```python
from build123d import *

# Parameters (mm, degrees)
SKETCH1_R           = 32.5
SKETCH1_R_2         = 2.3
SKETCH1_R_3         = 1.7
BOSS_EXTRUDE1_DEPTH = 5


with BuildPart() as part:
    # Sketch1 → Boss-Extrude1 (new body)
    with BuildSketch(Plane(origin=(0, 0, 0), x_dir=(1, 0, 0), z_dir=(0, 1, 0))):
        with Locations(Location((0, 0, 0), (0, 0, 270))):
            Circle(SKETCH1_R)
        with Locations(Location((-15, 20, 0), (0, 0, 270))):
            Circle(SKETCH1_R_2, mode=Mode.SUBTRACT)
        with Locations(Location((-22.5, 15, 0), (0, 0, 270))):
            Circle(SKETCH1_R_3, mode=Mode.SUBTRACT)
        with Locations(Location((-15, -20, 0), (0, 0, 270))):
            Circle(SKETCH1_R_2, mode=Mode.SUBTRACT)
        with Locations(Location((-25, 0, 0), (0, 0, 270))):
            Circle(SKETCH1_R_2, mode=Mode.SUBTRACT)
        with Locations(Location((-22.5, -15, 0), (0, 0, 270))):
            Circle(SKETCH1_R_3, mode=Mode.SUBTRACT)
        with Locations(Location((15, -20, 0), (0, 0, 90))):
            Circle(SKETCH1_R_2, mode=Mode.SUBTRACT)
        with Locations(Location((22.5, -15, 0), (0, 0, 90))):
            Circle(SKETCH1_R_3, mode=Mode.SUBTRACT)
        with Locations(Location((25, 0, 0), (0, 0, 90))):
            Circle(SKETCH1_R_2, mode=Mode.SUBTRACT)
        with Locations(Location((22.5, 15, 0), (0, 0, 90))):
            Circle(SKETCH1_R_3, mode=Mode.SUBTRACT)
        with Locations(Location((15, 20, 0), (0, 0, 90))):
            Circle(SKETCH1_R_2, mode=Mode.SUBTRACT)
        with BuildLine():
            Line((-9, 6.168261928), (-9, -16.9))
            Line((-9, -16.9), (9, -16.9))
            Line((9, -16.9), (9, 6.168261928))
            ThreePointArc((9, 6.168261928), (0, 19.3), (-9, 6.168261928))
        make_face(mode=Mode.SUBTRACT)
        with BuildLine():
            ThreePointArc((7.695243167, 22.633068138), (10.866931862, 24.195243167), (9.304756833, 27.366931862))
            ThreePointArc((9.304756833, 27.366931862), (0, 28.905491853), (-9.304756833, 27.366931862))
            ThreePointArc((-9.304756833, 27.366931862), (-10.866931862, 24.195243167), (-7.695243167, 22.633068138))
            ThreePointArc((-7.695243167, 22.633068138), (0, 23.905491853), (7.695243167, 22.633068138))
        make_face(mode=Mode.SUBTRACT)
        with BuildLine():
            ThreePointArc((7.695243167, -22.633068138), (10.866931862, -24.195243167), (9.304756833, -27.366931862))
            ThreePointArc((9.304756833, -27.366931862), (0, -28.905491853), (-9.304756833, -27.366931862))
            ThreePointArc((-9.304756833, -27.366931862), (-10.866931862, -24.195243167), (-7.695243167, -22.633068138))
            ThreePointArc((-7.695243167, -22.633068138), (0, -23.905491853), (7.695243167, -22.633068138))
        make_face(mode=Mode.SUBTRACT)
    extrude(amount=BOSS_EXTRUDE1_DEPTH)


solid = part.part
```
Source: CAD feature listing. Evaluate the final solid. Frame: model axes, mm. Give positions to 0.01 mm unless a question says otherwise; leave off trailing zeros. Order: outer loops, then holes, each group sorted by start corner. A loop starts at its lowest first (then second) coordinate and runs counter-clockwise, first axis right, second up.
(1) Section query C-C (x = -1.5). Return the cut outline in (y, z), plus the area to 3 significant figures.
(2) Contact query for flat-ended pins moving along their axis: P1, Ø4, axis at x = 15, z = -20, coming from the +Y side; P2, Ø2.5, axis at y = 1.5, z = 0, coming from the +X side; P3, Ø1.5, axis at y = 2.5, z = 3, coming from the -X side; P4, Ø1, axis at x = 17, y = 1, coming from the -Z side. Output: stop coordinate, or through.
(3) Pull-direction query (Z, two-part tool) for faces 1 (the face through (9, 2, 6)), 2 (the face through (9.76, 2.46, 31)), 3 (the face through (-14, 0, 0)); classes: +Z half, -Z half, draft (parallel to the pull), parting line (faces both ways), or undercut.
(4) Material intervals for line 1 along X through (y, z) = (2.15, 0); line 2 along Z through (x, y) = (1.5, 2.45); line 3 along Z through (x, y) = (7.5, 4.25), sorted ascending.
(5) Section query A-A (y = 3.25). State how many separate pieces and enclosed holes the cut face has, plus the area to 3 significant figures.
(6) Section query D-D (z = -9.65). Return the cut outline in (x, y).
(7) Section query B-B (z = 0). Return the cut outline in (x, y).
Outcome:
1. outline: (0, -32.47) - (5, -32.47) - (5, -28.87) - (0, -28.87) - close; (0, -23.86) - (5, -23.86) - (5, -19.18) - (0, -19.18) - close; (0, 16.9) - (5, 16.9) - (5, 23.86) - (0, 23.86) - close; (0, 28.87) - (5, 28.87) - (5, 32.47) - (0, 32.47) - close
1. area: 94.2 mm2
2. P1: passes through
2. P2: stops at x = 32.5
2. P3: stops at x = -32.42
2. P4: stops at z = -28
3. face 1: undercut
3. face 2: parting line
3. face 3: draft
4. line 1: x = -32.5 to -27.3, -22.7 to -9, 9 to 22.7, 27.3 to 32.5
4. line 2: z = -32.47 to -28.87, -23.86 to -19.18, 16.9 to 23.86, 28.87 to 32.47
4. line 3: z = -31.62 to -27.92, -22.7 to -15.72, 16.9 to 22.7, 27.92 to 31.62
5. separate pieces: 1
5. enclosed holes: 13
5. area: 2,340 mm2
6. outline: (-31.03, 0) - (-9.65, 0) - (-9.65, 5) - (-31.03, 5) - close; (9.65, 0) - (31.03, 0) - (31.03, 5) - (9.65, 5) - close
7. outline: (-32.5, 0) - (-27.3, 0) - (-27.3, 5) - (-32.5, 5) - close; (-22.7, 0) - (-9, 0) - (-9, 5) - (-22.7, 5) - close; (9, 0) - (22.7, 0) - (22.7, 5) - (9, 5) - close; (27.3, 0) - (32.5, 0) - (32.5, 5) - (27.3, 5) - close
